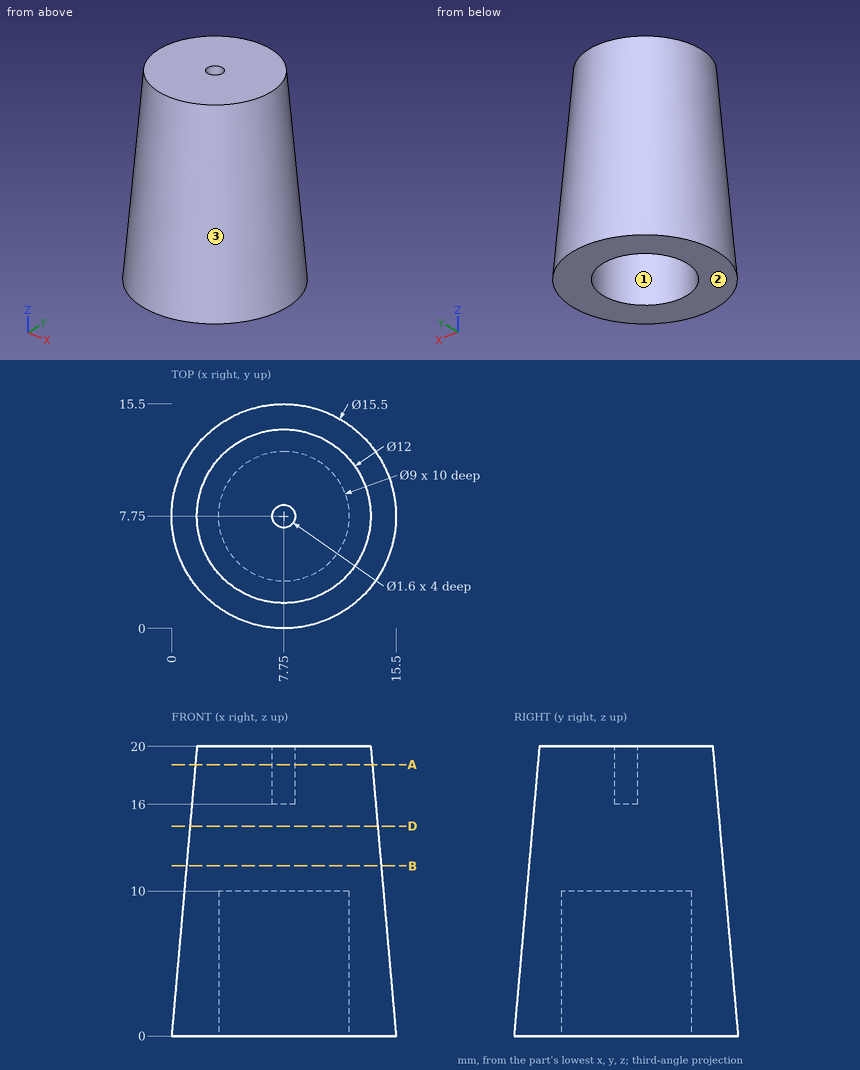
Design review of the part shown in the three views and the two pictorial views. Dimensions are in mm from the part's minimum x, y and z. Give positions to 0.01 mm unless a question says otherwise; leave off trailing zeros. Loops run counter-clockwise (first coordinate to the right, second up) from the corner with the lowest first, then second, coordinate; pieces in that order, holes last. Notation, with made-up numbers: (-7, -1) - (12, -1) arc R33 ccw to (12, 35) - close; hole circle Ø3 at (56, 55.5). An arc over 180 degrees is marked (long way). Answer as a JSON object with one key per item and string values.
Q1. Add section A-A on z = 18.75. State the section outline as (x, y) points, plus the area to 3 significant figures.
Worked out:
{"outline": "circle Ø12.22 at (7.75, 7.75); hole circle Ø1.6 at (7.75, 7.75)", "area": "115 mm^2"}
Q2. Mouldability with a two-part tool opening along Y and no side actions: class the marked faces 1, 2 and 3 as +Y half, -Y half, draft (parallel to the pull), parting line (faces both ways), or undercut.
Worked out:
{"face 1": "undercut", "face 2": "draft", "face 3": "parting line"}
Q3. Add section D-D on z = 14.5. State the section outline as (x, y) points, plus the area to 3 significant figures.
Worked out:
{"outline": "circle Ø12.96 at (7.75, 7.75)", "area": "132 mm^2"}
Q4. Add section B-B on z = 11.75. State the section outline as (x, y) points.
Worked out:
{"outline": "circle Ø13.44 at (7.75, 7.75)"}
Q5. To check wall thickness, follow line 1 along X through (y, z) = (9.25, 1.5); line 2 along Y through (x, z) = (11, 1); line 3 along Y through (x, z) = (7.25, 6). State the ranges of each line that lie inside material, in increasing order.
Worked out:
{"line 1": "x = 0.28 to 3.51, 11.99 to 15.22", "line 2": "y = 0.81 to 4.64, 10.86 to 14.69", "line 3": "y = 0.54 to 3.28, 12.22 to 14.96"}
Q6. Insertion check: pin 1 (6 mm diameter, centred on x = 14, z = 4, fed in from -Y); pin 2 (1.5 mm diameter, centred on x = 5, z = 8.5, fed in from -Y) (1 decimal); pin 3 (0.5 mm diameter, centred on x = 7.5, y = 8, fed in from +Z). Each pin has a flat end and moves straight along its axis. Give the tip position at first contact, or say it passes through.
Worked out:
{"pin 1": "stops at y = 1.07", "pin 2": "stops at y = 1", "pin 3": "stops at z = 16"}
